Work out the finished part from the listing and answer in its coordinate system (mm). Give positions to 0.01 mm unless a question says otherwise; leave off trailing zeros. Loops run counter-clockwise (first coordinate to the right, second up) from the corner with the lowest first, then second, coordinate; pieces in that order, holes last. Notation, with made-up numbers: (61, 36) - (99, 36) arc R33 ccw to (99, 65) - close; hole circle Ø1 at (52.25, -33.75). An arc over 180 degrees is marked (long way). One line per question, with ' | ' between items. Start each with the question number.
1. Section A-A (z = 89) is taken. Determine the outline of the cut face in (x, y).
2. Find the intervals of material crossed by line 1 (X direction, y = -1.35, z = -163); line 2 (X direction, y = -1.4, z = -86.5); line 3 (Y direction, x = -2, z = 337), in increasing order.
3. Each of these flat-tipped pins is pushed along its axis until it touches: pin 1 (3.5 mm diameter, centred on x = 0.97, z = 25.4, fed in from +Y); pin 2 (4.5 mm diameter, centred on x = 0.97, z = -25.4, fed in from -Y); pin 3 (1 mm diameter, centred on y = 1, z = -301.5, fed in from -X). Where does it stop, or does it pass through?
from build123d import *

# Parameters (mm, degrees)
BOSS_EXTRUDE1_START = -387.35
BOSS_EXTRUDE1_DEPTH = 774.7
SKETCH2_R           = 1.9812
CUT_EXTRUDE1_DEPTH  = 388.419680715
LPATTERN1_COUNT     = 16
LPATTERN1_PITCH     = 50.8


# Read off the part's stored shape, not the designer's step: Boss-Extrude1
with BuildPart() as part:
    # Boss-Extrude1 outline → Boss-Extrude1 (new body)
    with BuildSketch(Plane.XY.offset(BOSS_EXTRUDE1_START)):
        with BuildLine():
            ThreePointArc((-4.871384633, 1.524), (-5.01718702, 1.494998102), (-5.140792316, 1.412407684))
            Line((-5.140792316, 1.412407684), (-6.124107684, 0.429092316))
            ThreePointArc((-6.124107684, 0.429092316), (-6.206698102, 0.30548702), (-6.2357, 0.159684633))
            Line((-6.2357, 0.159684633), (-6.2357, -0.159684633))
            ThreePointArc((-6.2357, -0.159684633), (-6.206698102, -0.30548702), (-6.124107684, -0.429092316))
            Line((-6.124107684, -0.429092316), (-4.302592316, -2.250607684))
            ThreePointArc((-4.302592316, -2.250607684), (-4.17898702, -2.333198102), (-4.033184633, -2.3622))
            Line((-4.033184633, -2.3622), (-2.921, -2.3622))
            ThreePointArc((-2.921, -2.3622), (-2.651592316, -2.250607684), (-2.54, -1.9812))
            Line((-2.54, -1.9812), (-2.54, -1.27))
            ThreePointArc((-2.54, -1.27), (-2.311529276, -1.017286217), (-2.037131842, -1.2192))
            ThreePointArc((-2.037131842, -1.2192), (-1.904795163, -1.438121331), (-1.663829605, -1.524))
            Line((-1.663829605, -1.524), (4.871384633, -1.524))
            ThreePointArc((4.871384633, -1.524), (5.01718702, -1.494998102), (5.140792316, -1.412407684))
            Line((5.140792316, -1.412407684), (6.124107684, -0.429092316))
            ThreePointArc((6.124107684, -0.429092316), (6.206698102, -0.30548702), (6.2357, -0.159684633))
            Line((6.2357, -0.159684633), (6.2357, 0.159684633))
            ThreePointArc((6.2357, 0.159684633), (6.206698102, 0.30548702), (6.124107684, 0.429092316))
            Line((6.124107684, 0.429092316), (5.140792316, 1.412407684))
            ThreePointArc((5.140792316, 1.412407684), (5.01718702, 1.494998102), (4.871384633, 1.524))
            Line((4.871384633, 1.524), (-4.871384633, 1.524))
        make_face()
    extrude(amount=BOSS_EXTRUDE1_DEPTH)

    # Sketch2 → Cut-Extrude1 (cut, through all)
    with BuildSketch(Plane(origin=(0, 1.524, 0), x_dir=(1, 0, 0), z_dir=(0, 1, 0))):
        with Locations(Location((0.9652, -381, 0), (0, 0, 180))):
            Circle(SKETCH2_R)
    cut_extrude1 = extrude(amount=-CUT_EXTRUDE1_DEPTH, mode=Mode.SUBTRACT)

    # LPattern1: Cut-Extrude1 ×16
    with Locations(*[(0, 0, -i * LPATTERN1_PITCH) for i in range(1, LPATTERN1_COUNT)]):
        add(cut_extrude1, mode=Mode.SUBTRACT)


solid = part.part
Conclusion:
1) outline: (-6.24, -0.16) arc R0.38 ccw to (-6.12, -0.43) - (-4.3, -2.25) arc R0.38 ccw to (-4.03, -2.36) - (-2.92, -2.36) arc R0.38 ccw to (-2.54, -1.98) - (-2.54, -1.27) arc R0.25 cw to (-2.04, -1.22) arc R0.38 ccw to (-1.66, -1.52) - (4.87, -1.52) arc R0.38 ccw to (5.14, -1.41) - (6.12, -0.43) arc R0.38 ccw to (6.24, -0.16) - (6.24, 0.16) arc R0.38 ccw to (6.12, 0.43) - (5.14, 1.41) arc R0.38 ccw to (4.87, 1.52) - (-4.87, 1.52) arc R0.38 ccw to (-5.14, 1.41) - (-6.12, 0.43) arc R0.38 ccw to (-6.24, 0.16) - close
2) line 1: -5.2 to -2.54, -1.98 to 5.2 | line 2: -5.15 to -2.54, -1.95 to 5.15 | line 3: -1.32 to 1.52
3) pin 1: through | pin 2: y = -1.52 | pin 3: x = -6.05
